Part model, mm, in its own coordinate system. A direction names the side the tool comes from. Give positions to 0.01 mm unless a question says otherwise; leave off trailing zeros. Order: outer loops, then holes, each group sorted by start corner. A loop starts at its lowest first (then second) coordinate and runs counter-clockwise, first axis right, second up. Notation, with made-up numbers: (34.5, -25) - (66.5, -25) arc R37 cw to (66.5, 11) - close; hole circle Ø5 at (34, 67.25). An arc over 180 degrees is marked (long way). Use one line per item in the form item = value. Start each with the question number.
1. Band-saw the part on B-B, the plane z = 0. List the corners of the cut face in (x, y), plus the area to 3 significant figures.
2. Band-saw the part on A-A, the plane x = 0. List the corners of the cut face in (y, z), plus the area to 3 significant figures.
3. Pull direction Y, two halves, no side cores. Call faces 6 (the face through (-3.685, -10.879, -5.986)), 7 (the face through (-2, 0, 5)), 8 (the face through (-1, -9, 5.5)), 9 (the face through (-7.5, -7, -2)): +Y half, -Y half, draft (parallel to the pull), parting line (faces both ways), or undercut.
4. Tool access for faces 1 (the face through (7.5, -2, 0)), 2 (the face through (-5.5, -5, 0)), 3 (the face through (1.617, -13.986, -0.67)), 4 (the face through (-4.995, -7.72, 5.159)), 5 (the face through (0, -13, -2)): list every direction of +Z, -Z, +X, -X, +Y, -Y with a clear straight run to the whole face (end or side of a thin tool).
5. Drill centre lines: line 1 (X direction, y = -2.15, z = 0); line 2 (Z direction, x = 0, y = -14.25); line 3 (X direction, y = -7.5, z = 6.7). Where is each one in solid material? Low to high.
6. Band-saw the part on C-C, the plane y = -11.5. List the corners of the cut face in (x, z), plus the area to 3 significant figures.
7. Pin check, flat tips, straight feed: P1, Ø5.5, axis at y = -7.5, z = 0, coming from the +X side; P2, Ø9, axis at x = 0, y = -7.5, coming from the -Z side; P3, Ø5.5, axis at x = 0, z = 0, coming from the +Y side. Stop position of each tip, or through.
8. Band-saw the part on D-D, the plane x = 3.75. List the corners of the cut face in (y, z), plus the area to 3 significant figures.
from build123d import *

# Parameters (mm, degrees)
F0_W     = 15
F0_H     = 15
F0_R     = 1.75
F1_DEPTH = 15
F2_R     = 5
F3_DEPTH = 13
F4_R     = 1.75
F5_DEPTH = 15
F4_R_2   = 5
F6_DEPTH = 13
F7_R     = 1.65
F8_DEPTH = 15
F7_R_2   = 5
F9_DEPTH = 13


with BuildPart() as f1:
    # F0 (on Front) → F1 (new body)
    with BuildSketch(Plane.XZ):
        Rectangle(F0_W, F0_H)
        Circle(F0_R, mode=Mode.SUBTRACT)
    extrude(amount=F1_DEPTH)

    # F2 (on face) → F3 (cut)
    with BuildSketch(Plane.XZ):
        Circle(F2_R)
    extrude(amount=F3_DEPTH, mode=Mode.SUBTRACT)

    # F4 (on face) → F5 (cut)
    with BuildSketch(Plane.YZ.offset(7.5)):
        with Locations((-7.5, 0)):
            Circle(F4_R)
    extrude(amount=-F5_DEPTH, mode=Mode.SUBTRACT)

    # F4 (on face) → F6 (cut)
    with BuildSketch(Plane.YZ.offset(7.5)):
        with Locations((-7.5, 0)):
            Circle(F4_R_2)
        with Locations((-7.5, 0)):
            Circle(F4_R, mode=Mode.SUBTRACT)
    extrude(amount=-F6_DEPTH, mode=Mode.SUBTRACT)

    # F7 (on face) → F8 (cut)
    with BuildSketch(Plane(origin=(0, 0, -7.5), x_dir=(1, 0, 0), z_dir=(0, 0, -1))):
        with Locations((0, 7.5)):
            Circle(F7_R)
    extrude(amount=-F8_DEPTH, mode=Mode.SUBTRACT)

    # F7 (on face) → F9 (cut)
    with BuildSketch(Plane(origin=(0, 0, -7.5), x_dir=(1, 0, 0), z_dir=(0, 0, -1))):
        with Locations((0, 7.5)):
            Circle(F7_R_2)
        with Locations((0, 7.5)):
            Circle(F7_R, mode=Mode.SUBTRACT)
    extrude(amount=-F9_DEPTH, mode=Mode.SUBTRACT)


solid = f1.part
From the geometry:
q1.outline = (-7.5, -15) - (-1.75, -15) - (-1.75, -13) - (-5, -13) - (-5, -12.5) - (-5.5, -12.5) - (-5.5, -9.25) - (-7.5, -9.25) - close; (-7.5, -5.75) - (-5.5, -5.75) - (-5.5, -2.5) - (-5, -2.5) - (-5, 0) - (-7.5, 0) - close; (1.75, -15) - (7.5, -15) - (7.5, -12.5) - (5, -12.5) - (5, -13) - (1.75, -13) - close; (5, -2.5) - (7.5, -2.5) - (7.5, 0) - (5, 0) - close
q1.area = 51.0 mm²
q2.outline = (-15, -7.5) - (-12.5, -7.5) - (-12.5, -5) - (-13, -5) - (-13, -1.75) - (-15, -1.75) - close; (-15, 1.75) - (-13, 1.75) - (-13, 5) - (-12.5, 5) - (-12.5, 5.5) - (-9.15, 5.5) - (-9.15, 7.5) - (-15, 7.5) - close; (-5.85, 5.5) - (-2.5, 5.5) - (-2.5, 5) - (0, 5) - (0, 7.5) - (-5.85, 7.5) - close; (-2.5, -7.5) - (0, -7.5) - (0, -5) - (-2.5, -5) - close
q2.area = 51.4 mm²
q3.face_6 = undercut
q3.face_7 = +Y half
q3.face_8 = undercut
q3.face_9 = draft
q4.face_1 = +Z, -Z, +X, +Y, -Y
q4.face_2 = +X
q4.face_3 = +Y, -Y
q4.face_4 = -Z
q4.face_5 = +Y
q5.line_1 = -7.5 to -5, 5 to 7.5
q5.line_2 = -7.5 to -1.75, 1.75 to 7.5
q5.line_3 = -7.5 to -1.65, 1.65 to 7.5
q6.outline = (-7.5, -7.5) - (-3, -7.5) - (-3, -4) arc R5 cw to (-4, -3) - (-5.5, -3) - (-5.5, 3) - (-4, 3) arc R5 cw to (-3, 4) - (-3, 5.5) - (3, 5.5) - (3, 4) arc R5 cw to (4, 3) - (7.5, 3) - (7.5, 7.5) - (-7.5, 7.5) - close; (3, -7.5) - (7.5, -7.5) - (7.5, -3) - (4, -3) arc R5 cw to (3, -4) - close
q6.area = 103 mm²
q7.P1 = -5.5
q7.P2 = 5.5
q7.P3 = -13
q8.outline = (-15, -7.5) - (-10.81, -7.5) - (-10.81, -3.75) arc R5 cw to (-11.25, -3.31) - (-13, -3.31) - (-13, 3.31) - (-11.25, 3.31) arc R5 cw to (-10.81, 3.75) - (-10.81, 5.5) - (-4.19, 5.5) - (-4.19, 3.75) arc R5 cw to (-3.75, 3.31) - (0, 3.31) - (0, 7.5) - (-15, 7.5) - close; (-4.19, -7.5) - (0, -7.5) - (0, -3.31) - (-3.75, -3.31) arc R5 cw to (-4.19, -3.75) - close
q8.area = 96.4 mm²
